```python
from build123d import *

# Parameters (mm, degrees)
SKETCH1_W          = 10
SKETCH1_H          = 20
SKETCH2_R          = 5
CUT_EXTRUDE5_DEPTH = 5
CUT_EXTRUDE6_DEPTH = 15


with BuildPart() as part:
    # Sketch1 → Revolve1 (revolve)
    with BuildSketch(Plane.XY):
        with Locations((5, 10)):
            Rectangle(SKETCH1_W, SKETCH1_H)
    revolve(axis=Axis((0, 0, 0), (0, 1, 0)))

    # Sketch2 → Cut-Extrude5 (cut)
    with BuildSketch(Plane(origin=(0, 20, 0), x_dir=(1, 0, 0), z_dir=(0, 1, 0))):
        Circle(SKETCH2_R)
    extrude(amount=-CUT_EXTRUDE5_DEPTH, mode=Mode.SUBTRACT)

    # Sketch5 → Cut-Extrude6 (cut)
    with BuildSketch(Plane(origin=(0, 20, 0), x_dir=(1, 0, 0), z_dir=(0, 1, 0))):
        with BuildLine():
            Line((-10, 0), (-5, 0))
            ThreePointArc((-5, 0), (0, -5), (5, 0))
            Line((5, 0), (10, 0))
            ThreePointArc((10, 0), (0, -10), (-10, 0))
        make_face()
    extrude(amount=-CUT_EXTRUDE6_DEPTH, mode=Mode.SUBTRACT)


solid = part.part
```
Source: CAD feature listing. Evaluate the final solid. Frame: model axes, mm. A direction names the side the tool comes from. Coordinates: 2 decimals unless noted, no trailing zeros. Write each loop counter-clockwise with the first axis right and the second up, starting at its lowest first coordinate (ties: lowest second). Pieces come first, ordered by that corner, then holes. Notation, with made-up numbers: (5.5, 13) - (26.5, 13) arc R33 cw to (26.5, 48) - close; hole circle Ø4 at (-6.5, -18). An arc over 180 degrees is marked (long way). Answer as a JSON object with one key per item and string values.
Q1. Section query D-D, the plane x = -6. Output: boundary loops of the cut face in (y, z), plus the area to 3 significant figures.
Ans:
{"outline": "(0, -8) - (20, -8) - (20, 0) - (5, 0) - (5, 8) - (0, 8) - close", "area": "200 mm2"}
Q2. Section query C-C, the plane y = 11. Output: boundary loops of the cut face in (x, z).
Ans:
{"outline": "(-10, 0) arc R10 ccw to (10, 0) - (5, 0) arc R5 ccw to (-5, 0) - close"}
Q3. Material intervals for line 1 (Y direction, x = -7.5, z = 3.75); line 2 (Y direction, x = 0.25, z = -4.5); line 3 (X direction, y = 9.75, z = -0.25), sorted ascending. Write a range as [from, to].
Ans:
{"line 1": "y = [0, 5]", "line 2": "y = [0, 15]", "line 3": "x = [-10, 10]"}
Q4. Set-up query: faces 1 (the flat face through (0, 5, 6)), 2 (the cylindrical face through (-1.302, 7.918, -9.915)), 3 (the flat face through (7, 13, 0)). Return all of +Z, -Z, +X, -X, +Y, -Y with unobstructed straight access to the full face (end or side cutting, diameter ignored); none if empty.
Ans:
{"face 1": "+Z, +Y", "face 2": "+Y, -Y", "face 3": "+Z, +X, +Y"}
Q5. First-contact query: pin 1 Ø3 at (x, z) = (0, 0.5) entering from +Y; pin 2 Ø10 at (y, z) = (6.5, 5) entering from -X; pin 3 Ø1 at (x, y) = (-6, 4.5) entering from -Z. Flat tips, straight axial feed; report the tip coordinate or a pass-through.
Ans:
{"pin 1": "stops at y = 15", "pin 2": "stops at x = -10", "pin 3": "stops at z = -8.35"}
Q6. Draft query along X for faces 4 (the flat face through (-8, 13, 0)), 5 (the cylindrical face through (0, 18, -5)), 6 (the flat face through (0, 15, 0)), 7 (the cylindrical face through (0, 10, 5)). Return one class per face: released by +X, released by -X, zero draft, split by the parting line, or undercut.
Ans:
{"face 4": "zero draft", "face 5": "undercut", "face 6": "undercut", "face 7": "split by the parting line"}
Q7. Section query B-B, the plane z = 4. Output: boundary loops of the cut face in (x, y).
Ans:
{"outline": "(-9.17, 0) - (9.17, 0) - (9.17, 5) - (3, 5) - (3, 15) - (-3, 15) - (-3, 5) - (-9.17, 5) - close"}
Q8. Section query A-A, the plane x = 0. Output: boundary loops of the cut face in (y, z), plus the area to 3 significant figures.
Ans:
{"outline": "(0, -10) - (20, -10) - (20, -5) - (15, -5) - (15, 5) - (5, 5) - (5, 10) - (0, 10) - close", "area": "275 mm2"}
